Check sheet for the modelled part. Datum: model origin and axes. Units: mm. Round coordinates to 2 decimals unless told otherwise and drop trailing zeros. Order: outer loops, then holes, each group sorted by start corner. A loop starts at its lowest first (then second) coordinate and runs counter-clockwise, first axis right, second up.
Autodesk Inventor part; units mm, degrees
ref_plane "Work Plane1" through (-273.6, -145.5093, 1.1) normal (0, 0, 1) x (1, 0, 0)
ref_plane "YZ Plane" through (0, 0, 0) normal (1, 0, 0) x (0, 1, 0)
ref_plane "XZ Plane" through (0, 0, 0) normal (0, 1, 0) x (-1, 0, 0)
ref_plane "Work Plane1" through (-273.6, -145.5093, 1.1) normal (0, 0, 1) x (1, 0, 0)
sketch "Sketch1" plane through (0, 0, 0) normal (0, 0, 1) x (1, 0, 0)
  line L0 (-273.6, -142.1074) -> (-273.6, 15)
  line L1 (-273.6, -142.1074) -> (-273.5328, -142.3023)
  line L2 (-273.5328, -142.3023) -> (-271.5577, -145.5093)
  line L3 (-271.5577, -145.5093) -> (27.9577, -145.5093)
  line L4 (27.9577, -145.5093) -> (29.9328, -142.3023)
  line L5 (29.9328, -142.3023) -> (30, -142.1074)
  line L6 (30, -142.1074) -> (30, 15)
  line L7 (30, 15) -> (-273.6, 15)
  ellipse E0 centre (-207.1368, -126.3725) end of major axis (-207.1368, -124.9133) minor radius 1.45 (-205.7085, -126.6236) -> (-208.5652, -126.6236) ccw
  ellipse E1 centre (-207.1368, -126.8715) end of major axis (-205.6868, -126.8715) minor radius 1.4408 (-208.5652, -126.6236) -> (-205.7085, -126.6236) ccw
  line L8 (10, -5) -> (-10, -5)
  line L9 (-10, -5) -> (-10, 5)
  line L10 (-10, 5) -> (10, 5)
  line L11 (10, 5) -> (10, -5)
  line L12 (-131.8, -134.6879) -> (-131.8, -124.6879)
  line L13 (-131.8, -124.6879) -> (-111.8, -124.6879)
  line L14 (-111.8, -124.6879) -> (-111.8, -134.6879)
  line L15 (-111.8, -134.6879) -> (-131.8, -134.6879)
  line L16 (-233.6, -124.6879) -> (-233.6, -134.6879)
  line L17 (-233.6, -134.6879) -> (-253.6, -134.6879)
  line L18 (-253.6, -134.6879) -> (-253.6, -124.6879)
  line L19 (-253.6, -124.6879) -> (-233.6, -124.6879)
  line L20 (-131.8, -5) -> (-131.8, 5)
  line L21 (-131.8, 5) -> (-111.8, 5)
  line L22 (-111.8, 5) -> (-111.8, -5)
  line L23 (-111.8, -5) -> (-131.8, -5)
  line L24 (-10, -124.6879) -> (10, -124.6879)
  line L25 (10, -124.6879) -> (10, -134.6879)
  line L26 (10, -134.6879) -> (-10, -134.6879)
  line L27 (-10, -134.6879) -> (-10, -124.6879)
  line L28 (-233.6, 5) -> (-233.6, -5)
  line L29 (-233.6, -5) -> (-253.6, -5)
  line L30 (-253.6, -5) -> (-253.6, 5)
  line L31 (-253.6, 5) -> (-233.6, 5)
  ellipse E2 centre (-268.2527, 10.0167) end of major axis (-268.2527, 11.4759) minor radius 1.45 (-266.8028, 9.9997) -> (-269.7026, 9.9997) ccw
  ellipse E3 centre (-268.2527, 9.9828) end of major axis (-268.2527, 8.5236) minor radius 1.45 (-269.7026, 9.9997) -> (-266.8028, 9.9997) ccw
  ellipse E4 centre (25.0696, -126.3725) end of major axis (25.0696, -124.9133) minor radius 1.45 (26.5195, -126.3895) -> (23.6197, -126.3895) ccw
  ellipse E5 centre (25.0696, -126.4064) end of major axis (25.0696, -127.8656) minor radius 1.45 (23.6197, -126.3895) -> (26.5195, -126.3895) ccw
  ellipse E6 centre (-268.2527, -58.2135) end of major axis (-268.2527, -56.7542) minor radius 1.45 (-266.8028, -58.2304) -> (-269.7026, -58.2304) ccw
  ellipse E7 centre (-268.2527, -58.2474) end of major axis (-268.2527, -59.7066) minor radius 1.45 (-269.7026, -58.2304) -> (-266.8028, -58.2304) ccw
  ellipse E8 centre (-83.992, 10.0167) end of major axis (-83.992, 11.4759) minor radius 1.45 (-82.5421, 9.9997) -> (-85.4419, 9.9997) ccw
  ellipse E9 centre (-83.992, 9.9828) end of major axis (-83.992, 8.5236) minor radius 1.45 (-85.4419, 9.9997) -> (-82.5421, 9.9997) ccw
  ellipse E10 centre (25.0696, -58.2135) end of major axis (25.0696, -56.7542) minor radius 1.45 (26.5195, -58.2304) -> (23.6197, -58.2304) ccw
  ellipse E11 centre (25.0696, -58.2474) end of major axis (25.0696, -59.7066) minor radius 1.45 (23.6197, -58.2304) -> (26.5195, -58.2304) ccw
  ellipse E12 centre (-62.1557, -126.3725) end of major axis (-62.1557, -124.9133) minor radius 1.45 (-60.7058, -126.3895) -> (-63.6056, -126.3895) ccw
  ellipse E13 centre (-62.1557, -126.4064) end of major axis (-62.1557, -127.8656) minor radius 1.45 (-63.6056, -126.3895) -> (-60.7058, -126.3895) ccw
  ellipse E14 centre (-268.2527, -126.3725) end of major axis (-268.2527, -124.9133) minor radius 1.45 (-266.8028, -126.3895) -> (-269.7026, -126.3895) ccw
  ellipse E15 centre (-268.2527, -126.4064) end of major axis (-268.2527, -127.8656) minor radius 1.45 (-269.7026, -126.3895) -> (-266.8028, -126.3895) ccw
  ellipse E16 centre (-167.7791, 10.0167) end of major axis (-167.7791, 11.4759) minor radius 1.45 (-166.3292, 9.9997) -> (-169.229, 9.9997) ccw
  ellipse E17 centre (-167.7791, 9.9828) end of major axis (-167.7791, 8.5236) minor radius 1.45 (-169.229, 9.9997) -> (-166.3292, 9.9997) ccw
  ellipse E18 centre (-151.1416, -126.3725) end of major axis (-151.1416, -124.9133) minor radius 1.45 (-149.7132, -126.6236) -> (-152.5699, -126.6236) ccw
  ellipse E19 centre (-151.1416, -126.8715) end of major axis (-149.6916, -126.8715) minor radius 1.4408 (-152.5699, -126.6236) -> (-149.7132, -126.6236) ccw
  ellipse E20 centre (25.0696, 10.0167) end of major axis (25.0696, 11.4759) minor radius 1.45 (26.5195, 9.9997) -> (23.6197, 9.9997) ccw
  ellipse E21 centre (25.0696, 9.9828) end of major axis (25.0696, 8.5236) minor radius 1.45 (23.6197, 9.9997) -> (26.5195, 9.9997) ccw
  line L32 (-9.8, 4.8) -> (9.8, 4.8)
  line L33 (9.8, 4.8) -> (9.8, -4.8)
  line L34 (9.8, -4.8) -> (-9.8, -4.8)
  line L35 (-9.8, -4.8) -> (-9.8, 4.8)
  line L36 (-6.8, 1.8) -> (6.8, 1.8)
  line L37 (6.8, 1.8) -> (6.8, -1.8)
  line L38 (6.8, -1.8) -> (-6.8, -1.8)
  line L39 (-6.8, -1.8) -> (-6.8, 1.8)
  point P0 (0, 0)
  point P1 (0, 0)
  point P2 (-121.8, 0)
  point P3 (-243.6, 0)
  point P4 (-243.6, -129.6879)
  point P5 (-121.8, -129.6879)
  point P6 (0, -129.6879)
  point P7 (0, 0)
  dimension "d0" = 19.6
  dimension "d1" = 9.6
  dimension "d2" = 13.6
  dimension "d3" = 3.6
extrude "Extrusion1" add sketch "Sketch1" along normal blind 1.3 contours L32 L33 L34 L35 | L36 L37 L38 L39
sketch "Sketch2" plane through (0, 0, 1.3) normal (0, 0, 1) x (1, 0, 0)
  line L0 (-6.8, 1.8) -> (6.8, 1.8)
  line L1 (6.8, 1.8) -> (6.8, -1.8)
  line L2 (6.8, -1.8) -> (-6.8, -1.8)
  line L3 (-6.8, -1.8) -> (-6.8, 1.8)
  point P0 (0, 0)
  point P1 (0, 0)
  dimension "d6" = 13.6
  dimension "d7" = 3.6
extrude "Extrusion2" add sketch "Sketch2" along normal blind 1.7
sketch "Sketch3" plane through (-9.8, -4.8, 0) normal (0, -1, 0) x (1, 0, 0)
  line L0 (16.6, 3) -> (3, 3)
  line L1 (0, 1.3) -> (3, 3)
  line L2 (3, 3) -> (16.6, 3)
  line L3 (19.6, 1.3) -> (0, 1.3)
  line L4 (16.6, 3) -> (19.6, 1.3)
  line L5 (0, 0) -> (0, 1.3)
  line L6 (19.6, 1.3) -> (0, 1.3)
  point P0 (9.8, 0)
extrude "Extrusion3" add sketch "Sketch3" against normal up to surface (9.6 mm away)
sketch "Sketch4" plane through (9.8, -4.8, 0) normal (1, 0, 0) x (0, 0, -1)
  line L0 (0, 0) -> (-1.3, 0)
  line L1 (-1.3, 0) -> (-1.3, 3)
  line L2 (-1.3, 9.6) -> (-1.3, 0)
  line L3 (0, 9.6) -> (-1.3, 9.6)
  line L4 (-1.3, 9.6) -> (-1.3, 6.6)
  line L5 (-1.3, 0) -> (-3, 3)
  line L6 (-3, 0) -> (-3, 9.6)
  line L7 (-3, 6.6) -> (-1.3, 9.6)
  line L8 (-3, 0) -> (-1.3, 0)
  line L9 (-1.3, 0) -> (-3, 0)
  line L10 (-3, 0) -> (-3, 9.6)
  line L11 (-3, 9.6) -> (-1.3, 9.6)
  line L12 (-3, 9.6) -> (-1.3, 9.6)
  point P0 (0, 4.8)
  dimension "d12" = 3
  dimension "d13" = 3
extrude "Extrusion4" cut sketch "Sketch4" against normal through all contours L8 L6 L5 | L6 L11 L7
properties part number "Pads"
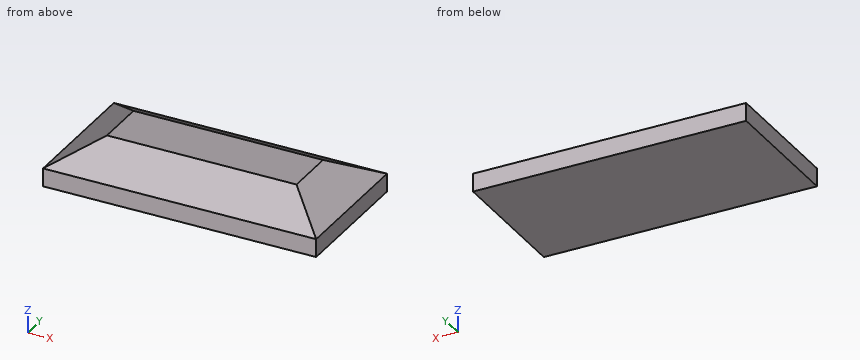
Item 1: Sectioned sample at A-A (x = 2). Record the cut outline in (y, z).
Answer:
outline: (-4.8, 0) - (4.8, 0) - (4.8, 1.3) - (1.8, 3) - (-1.8, 3) - (-4.8, 1.3) - close
Item 2: Sectioned sample at D-D (z = 1.5). Record the cut outline in (x, y), and give its area (3 significant figures).
Answer:
outline: (-9.45, -4.45) - (9.45, -4.45) - (9.45, 4.45) - (-9.45, 4.45) - close
area: 168 mm2
Item 3: Sectioned sample at B-B (y = 0). Record the cut outline in (x, z).
Answer:
outline: (-9.8, 0) - (9.8, 0) - (9.8, 1.3) - (6.8, 3) - (-6.8, 3) - (-9.8, 1.3) - close
Item 4: Sectioned sample at C-C (z = 2.5). Record the cut outline in (x, y).
Answer:
outline: (-7.68, -2.68) - (7.68, -2.68) - (7.68, 2.68) - (-7.68, 2.68) - close
Item 5: Scan lines: line 1 along Z through (x, y) = (7.75, 0.5); line 2 along X through (y, z) = (2, 2.75); line 3 along Z through (x, y) = (-2.25, -3.5). Record each from-to range of solid material in increasing order.
Answer:
line 1: z = 0 to 2.46
line 2: x = -7.24 to 7.24
line 3: z = 0 to 2.04
